CAD build for the part. Positions are in the model's coordinates, mm. Face numbers are marked on the shaded views. A direction names the side the tool comes from. Round coordinates to 2 decimals unless told otherwise and drop trailing zeros. Loops run counter-clockwise (first coordinate to the right, second up) from the corner with the lowest first, then second, coordinate; pieces in that order, holes last.
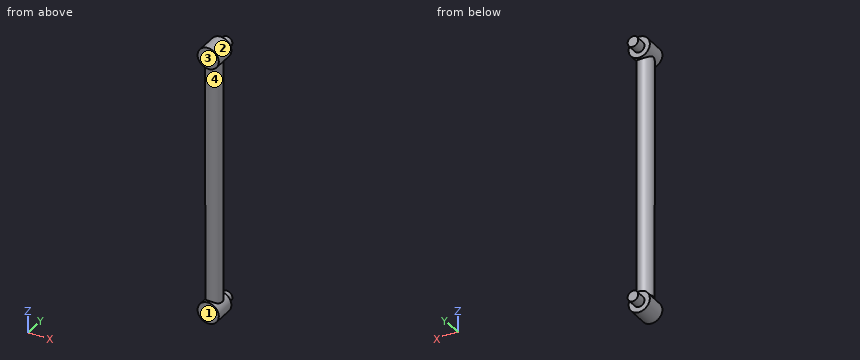
from build123d import *

# Parameters (mm, degrees)
SKIZZE1_R                       = 1.5
AUFSATZ_LINEAR_AUSTRAGEN1_DEPTH = 46
AUFSATZ_LINEAR_START            = -2
SKIZZE2_R                       = 2
AUFSATZ_LINEAR_AUSTRAGEN2_DEPTH = 4
SKIZZE3_R                       = 1
AUFSATZ_LINEAR_AUSTRAGEN4_DEPTH = 2


with BuildPart() as part:
    # Skizze1 → Aufsatz-Linear austragen1 (new body)
    with BuildSketch(Plane.XY):
        Circle(SKIZZE1_R)
    extrude(amount=AUFSATZ_LINEAR_AUSTRAGEN1_DEPTH)

    # Skizze2 → Aufsatz-Linear austragen2 (add)
    with BuildSketch(Plane(origin=(0, 0, 0), x_dir=(1, 0, 0), z_dir=(0, 1, 0)).offset(AUFSATZ_LINEAR_START)):
        with Locations((0, -47.23803597)):
            Circle(SKIZZE2_R)
        with Locations((0, 1.58182535)):
            Circle(SKIZZE2_R)
    extrude(amount=AUFSATZ_LINEAR_AUSTRAGEN2_DEPTH)

    # Skizze3 → Aufsatz-Linear austragen4 (add)
    with BuildSketch(Plane(origin=(0, 2, 0), x_dir=(1, 0, 0), z_dir=(0, 1, 0))):
        with Locations((0, -47.23803597)):
            Circle(SKIZZE3_R)
        with Locations((0, 1.58182535)):
            Circle(SKIZZE3_R)
    extrude(amount=AUFSATZ_LINEAR_AUSTRAGEN4_DEPTH)


solid = part.part
Item 1: Cut at C-C (z = 32). List the corners of the cut face in (x, y).
Verdict:
outline: circle Ø3 at (0, 0)
Item 2: Wall check: L1, parallel to Z at x = 0, y = 2.75; L2, parallel to X at y = 0, z = 32.5; L3, parallel to Z at x = -0.8, y = 2.75. Give the ranges that are in metal, low to high.
Verdict:
L1: z = -2.58 to -0.58, 46.24 to 48.24
L2: x = -1.5 to 1.5
L3: z = -2.18 to -0.98, 46.64 to 47.84
Item 3: Mould opens along Z. For the marked faces 1 and 2 say: released by +Z, released by -Z, zero draft, split by the parting line, or undercut.
Verdict:
face 1: zero draft
face 2: undercut
Item 4: Flat gauge pins, fed straight in: P1, Ø1.5, axis at x = 1.5, y = 2, coming from the -Z side; P2, Ø1, axis at y = 3, z = 34, coming from the +X side; P3, Ø2, axis at x = -1.5, y = -1, coming from the -Z side; P4, Ø1.2, axis at x = 1, z = -2.5, coming from the +Y side. Where does each tip first touch, or does it go through?
Verdict:
P1: stops at z = -3.44
P2: passes through
P3: stops at z = -3.52
P4: stops at y = 4
Item 5: Cut at A-A (x = 0). List the corners of the cut face in (y, z).
Verdict:
outline: (-2, -3.58) - (2, -3.58) - (2, -2.58) - (4, -2.58) - (4, -0.58) - (2, -0.58) - (2, 0.42) - (1.5, 0.42) - (1.5, 45.24) - (2, 45.24) - (2, 46.24) - (4, 46.24) - (4, 48.24) - (2, 48.24) - (2, 49.24) - (-2, 49.24) - (-2, 45.24) - (-1.5, 45.24) - (-1.5, 0.42) - (-2, 0.42) - close
Item 6: 3-axis set-ups, long thin cutter, end or side, ignore diameter. For the marked faces 3 and 4: which of +Z, -Z, +X, -X, +Y, -Y reach the whole face in a straight line?
Verdict:
face 3: +Z, -Z, +X, -X, -Y
face 4: none
Item 7: Cut at B-B (y = 0). List the corners of the cut face in (x, z).
Verdict:
outline: (-1.5, 0) - (-1.22, 0) arc R2 ccw (long way) to (1.22, 0) - (1.5, 0) - (1.5, 45.92) arc R2 ccw (long way) to (-1.5, 45.92) - close
